Work out the finished part from the listing and answer in its coordinate system (mm). A direction names the side the tool comes from. Round coordinates to 2 decimals unless told otherwise and drop trailing zeros. Order: outer loops, then holes, each group sorted by start corner. A loop starts at its lowest first (then second) coordinate and runs counter-clockwise, first axis right, second up. Notation, with made-up numbers: (17.5, 57.25) -> (66.5, 57.25) arc R31 cw to (66.5, 88.25) -> close; hole circle Ø9 at (56, -7). An arc over 180 degrees is marked (long way). Use a Markdown table: item, result. Add a question column.
Item 1: A cutting plane is placed at C-C, the plane y = 0. Determine the outline of the cut face in (x, z), plus the area to 3 significant figures.
Item 2: Flat-ended cylindrical pins translate along their axes: P1, Ø6, axis at x = -20.5, z = 35.5, coming from the -Y side; P2, Ø1, axis at x = -5.5, z = 35, coming from the +Y side; P3, Ø6, axis at x = -22, z = 34.5, coming from the +Y side; P4, Ø12, axis at x = 29.01, y = 0, coming from the -Z side. Find the tip coordinate at first contact, or state that the pin passes through.
Item 3: Find the intervals of material crossed by L1, parallel to Y at x = -13, z = 10; L2, parallel to Y at x = 22.5, z = 26.5; L3, parallel to X at y = -9, z = 14.5, in increasing order. Write a range as [from, to].
Item 4: A cutting plane is placed at D-D, the plane x = 24. Determine the outline of the cut face in (y, z), plus the area to 3 significant figures.
Item 5: A cutting plane is placed at B-B, the plane x = -28. Determine the outline of the cut face in (y, z), plus the area to 3 significant figures.
Item 6: For a pull along Y with two mould halves and no side action, classify faces 1 (the flat face through (-21, -27.475, 29)), 2 (the cylindrical face through (2.897, 40.522, 3.055)), 3 (the cylindrical face through (-2.9, 33.07, 29.66)) as +Y half, -Y half, draft (parallel to the pull), parting line (faces both ways), or undercut.
Item 7: A tool of negligible diameter and unlimited length cuts with its end or side. For faces 4 (the flat face through (22, 48.498, 29)), 5 (the cylindrical face through (-3.06, -32.91, 29.66)), from which of +Z, -Z, +X, -X, +Y, -Y can it reach the whole face along a straight path? Write none if from no direction.
from build123d import *

# Parameters (mm, degrees)
F0_W     = 40.881359
F0_H     = 60.0299
F1_DEPTH = 48.612542
F2_R     = 10.16
F3_T     = -2.54
F5_D     = 15.24


with BuildPart() as f1:
    # F0 (on Top) → F1 (new body)
    with BuildSketch(Plane.XY):
        Polygon((43.658987, 51.038296), (0, 51.038296), (0, 30.01495), (0, -30.01495), (0, -51.038296), (43.658987, -51.038296), align=None)
        with Locations((-20.440679, 0)):
            Rectangle(F0_W, F0_H)
    extrude(amount=F1_DEPTH)

    # F2
    f2_edges = [f1.edges().sort_by_distance(p)[0] for p in [
        (0, 51.038296, 24.306271),
        (43.658987, -51.038296, 24.306271),
        (43.658987, 51.038296, 24.306271),
        (0, -51.038296, 24.306271),
        (43.658987, 0, 0),
        (21.829493, 51.038296, 0),
        (0, 40.526623, 0),
        (-20.44068, 30.01495, 0),
        (-40.881359, 0, 0),
        (-20.44068, -30.01495, 0),
        (0, -40.526623, 0),
        (21.829493, -51.038296, 0),
        (0, 30.01495, 24.306271),
        (-40.881359, 30.01495, 24.306271),
        (-40.881359, -30.01495, 24.306271),
        (0, -30.01495, 24.306271),
    ]]
    fillet(f2_edges, radius=F2_R)

    # F3
    f3_openings = [f1.faces().sort_by_distance(p)[0] for p in [
        (6.859627, 0, 48.612542),
    ]]
    offset(amount=F3_T, openings=f3_openings)

    # F5 (through all)
    with Locations(Plane(origin=(0, 0, 0), x_dir=(1, 0, 0), z_dir=(0, 0, -1))):
        with Locations((29.013653, 0)):
            Hole(F5_D / 2)


solid = f1.part
Reported:
| question | item | result |
|---|---|---|
| 1 | outline | (-40.88, 10.16) arc R10.16 ccw to (-30.72, 0) -> (21.39, 0) -> (21.39, 2.54) -> (-30.72, 2.54) arc R7.62 cw to (-38.34, 10.16) -> (-38.34, 48.61) -> (-40.88, 48.61) -> close; (36.63, 0.5) arc R10.16 ccw to (43.66, 10.16) -> (43.66, 48.61) -> (41.12, 48.61) -> (41.12, 10.16) arc R7.62 cw to (36.63, 3.21) -> close |
| 1 | area | 391 mm² |
| 2 | P1 | y = -30.01 |
| 2 | P2 | y = 31.42 |
| 2 | P3 | y = 30.01 |
| 2 | P4 | through |
| 3 | L1 | [-30.01, -27.47], [27.47, 30.01] |
| 3 | L2 | [-51.04, -48.5], [48.5, 51.04] |
| 3 | L3 | [-40.88, -38.34], [41.12, 43.66] |
| 4 | outline | (-51.04, 10.16) arc R10.16 ccw to (-40.88, 0) -> (-5.74, 0) -> (-5.74, 2.54) -> (-40.88, 2.54) arc R7.62 cw to (-48.5, 10.16) -> (-48.5, 48.61) -> (-51.04, 48.61) -> close; (5.74, 0) -> (40.88, 0) arc R10.16 ccw to (51.04, 10.16) -> (51.04, 48.61) -> (48.5, 48.61) -> (48.5, 10.16) arc R7.62 cw to (40.88, 2.54) -> (5.74, 2.54) -> close |
| 4 | area | 445 mm² |
| 5 | outline | (-30.01, 10.16) arc R10.16 ccw to (-19.85, 0) -> (19.85, 0) arc R10.16 ccw to (30.01, 10.16) -> (30.01, 48.61) -> (27.47, 48.61) -> (27.47, 10.16) arc R7.62 cw to (19.85, 2.54) -> (-19.85, 2.54) arc R7.62 cw to (-27.47, 10.16) -> (-27.47, 48.61) -> (-30.01, 48.61) -> close |
| 5 | area | 367 mm² |
| 6 | face 1 | undercut |
| 6 | face 2 | draft |
| 6 | face 3 | +Y half |
| 7 | face 4 | +Z |
| 7 | face 5 | +Z, -Z, -X, -Y |
